Read the model definition and answer for the solid it produces. Units are mm, in the model's axes. A direction names the side the tool comes from. Coordinates: 2 decimals unless noted, no trailing zeros. Order: outer loops, then holes, each group sorted by start corner. A loop starts at its lowest first (then second) coordinate and runs counter-clockwise, first axis right, second up. Notation, with made-up numbers: M -11.75,33 L 23.25,33 A24 cw 23.25,53 Z; hole C -14.5,-18.75 d7. An arc over 180 degrees is marked long. Put each result on its own line as item: value.
from build123d import *

# Parameters (mm, degrees)
F0_R     = 1.6
F0_R_2   = 1.130501
F0_R_3   = 4.5
F0_R_4   = 5.5
F0_R_5   = 1.1305
F1_DEPTH = 1.6


with BuildPart() as f1:
    # F0 (on Top) → F1 (new body)
    with BuildSketch(Plane.XY):
        with BuildLine():
            Line((0, 6.68), (-4.5, 6.68))
            Line((-4.5, 6.68), (-4.5, 17.5))
            Line((-4.5, 17.5), (-10.717738, 23.909049))
            Line((-10.717738, 23.909049), (-12.710509, 25.963134))
            ThreePointArc((-12.710509, 25.963134), (-15.99118, 28.209543), (-19.887888, 29.000001))
            Line((-19.887888, 29.000001), (-27.5, 29.000001))
            ThreePointArc((-27.5, 29.000001), (-31.742641, 27.242641), (-33.5, 23.000001))
            Line((-33.5, 23.000001), (-33.5, 7))
            ThreePointArc((-33.5, 7), (-32.053216, 2.411389), (-28.236161, -0.517541))
            Line((-28.236161, -0.517541), (-21.823232, -2.851656))
            ThreePointArc((-21.823232, -2.851656), (-19.437572, -4.682237), (-18.533332, -7.550119))
            Line((-18.533332, -7.550119), (-18.533332, -8))
            Line((-18.533332, -8), (-18.533332, -8.449881))
            ThreePointArc((-18.533332, -8.449881), (-19.437572, -11.317763), (-21.823232, -13.148344))
            Line((-21.823232, -13.148344), (-28.236161, -15.482459))
            ThreePointArc((-28.236161, -15.482459), (-32.053216, -18.411389), (-33.5, -23))
            Line((-33.5, -23), (-33.5, -29.5))
            ThreePointArc((-33.5, -29.5), (-31.156854, -35.156854), (-25.5, -37.5))
            Line((-25.5, -37.5), (-20.777138, -37.5))
            ThreePointArc((-20.777138, -37.5), (-17.336651, -36.747083), (-14.525119, -34.625971))
            ThreePointArc((-14.525119, -34.625971), (-7.993173, -29.698059), (0, -27.94883))
            ThreePointArc((0, -27.94883), (7.993173, -29.698059), (14.525119, -34.625971))
            ThreePointArc((14.525119, -34.625971), (17.336651, -36.747083), (20.777138, -37.5))
            Line((20.777138, -37.5), (25.5, -37.5))
            ThreePointArc((25.5, -37.5), (31.156854, -35.156854), (33.5, -29.5))
            Line((33.5, -29.5), (33.5, -23))
            ThreePointArc((33.5, -23), (32.053216, -18.411389), (28.236161, -15.482459))
            Line((28.236161, -15.482459), (21.823232, -13.148344))
            ThreePointArc((21.823232, -13.148344), (19.437572, -11.317763), (18.533332, -8.449881))
            Line((18.533332, -8.449881), (18.533332, -8))
            Line((18.533332, -8), (18.533332, -7.550119))
            ThreePointArc((18.533332, -7.550119), (19.437572, -4.682237), (21.823232, -2.851656))
            Line((21.823232, -2.851656), (28.236161, -0.517541))
            ThreePointArc((28.236161, -0.517541), (32.053216, 2.411389), (33.5, 7))
            Line((33.5, 7), (33.5, 23.000001))
            ThreePointArc((33.5, 23.000001), (31.742641, 27.242641), (27.5, 29.000001))
            Line((27.5, 29.000001), (19.887888, 29.000001))
            ThreePointArc((19.887888, 29.000001), (15.99118, 28.209543), (12.710509, 25.963134))
            Line((12.710509, 25.963134), (10.717738, 23.909049))
            Line((10.717738, 23.909049), (4.5, 17.5))
            Line((4.5, 17.5), (4.5, 6.68))
            Line((4.5, 6.68), (0, 6.68))
        make_face()
        with Locations((-25.5, -33.5)):
            Circle(F0_R, mode=Mode.SUBTRACT)
        with Locations((-17.5, -30)):
            Circle(F0_R_2, mode=Mode.SUBTRACT)
        with Locations((-25.5, -23)):
            Circle(F0_R_3, mode=Mode.SUBTRACT)
        with Locations((-15.25, -23.25)):
            Circle(F0_R, mode=Mode.SUBTRACT)
        with Locations((15.25, -23.25)):
            Circle(F0_R, mode=Mode.SUBTRACT)
        with Locations((17.5, -30)):
            Circle(F0_R_2, mode=Mode.SUBTRACT)
        with Locations((25.5, -33.5)):
            Circle(F0_R, mode=Mode.SUBTRACT)
        with Locations((25.5, -23)):
            Circle(F0_R_3, mode=Mode.SUBTRACT)
        with Locations((0, -8)):
            Circle(F0_R_4, mode=Mode.SUBTRACT)
        with Locations((-25.5, 7)):
            Circle(F0_R_3, mode=Mode.SUBTRACT)
        with Locations((-15.25, 7.25)):
            Circle(F0_R, mode=Mode.SUBTRACT)
        with Locations((-25.5, 17.5)):
            Circle(F0_R, mode=Mode.SUBTRACT)
        with Locations((-17.500001, 16.5)):
            Circle(F0_R_5, mode=Mode.SUBTRACT)
        with Locations((-23.5, 24.000001)):
            Circle(F0_R_2, mode=Mode.SUBTRACT)
        with Locations((15.25, 7.25)):
            Circle(F0_R, mode=Mode.SUBTRACT)
        with Locations((25.5, 7)):
            Circle(F0_R_3, mode=Mode.SUBTRACT)
        with Locations((17.500001, 16.5)):
            Circle(F0_R_5, mode=Mode.SUBTRACT)
        with Locations((25.5, 17.5)):
            Circle(F0_R, mode=Mode.SUBTRACT)
        with Locations((23.5, 24.000001)):
            Circle(F0_R_2, mode=Mode.SUBTRACT)
    extrude(amount=F1_DEPTH)


solid = f1.part
Q1. Find section C-C on x = 15.5. Write down the section's boundary in (y, z).
Answers below:
outline: M -35.59,0 L -24.83,0 L -24.83,1.6 L -35.59,1.6 Z; M -21.67,0 L 5.67,0 L 5.67,1.6 L -21.67,1.6 Z; M 8.83,0 L 27.99,0 L 27.99,1.6 L 8.83,1.6 Z
Q2. Consider line 1 along X through (y, z) = (-26, 1.3); line 2 along X through (y, z) = (-21, 0.2); line 3 along Y through (x, z) = (15, 0.9). Determine where each line is inside the solid, lowest interval first.
Answers below:
line 1: x = -33.5 to -28.85, -22.15 to 22.15, 28.85 to 33.5
line 2: x = -33.25 to -29.53, -21.47 to 21.47, 29.53 to 33.25
line 3: y = -35.13 to -24.83, -21.67 to 5.67, 8.83 to 27.72
Q3. Find section A-A on x = -2.5. Write down the section's boundary in (y, z), plus the area to 3 significant figures.
Answers below:
outline: M -28.11,0 L -12.9,0 L -12.9,1.6 L -28.11,1.6 Z; M -3.1,0 L 6.68,0 L 6.68,1.6 L -3.1,1.6 Z
area: 40.0 mm^2
Q4. Given pin 1 (14.5 mm diameter, centred on x = -25.5, y = 7, fed in from +Z), flat-ended and moving along its own axis, determine where the tip first touches the part or whether it passes through.
Answers below:
pin 1: stops at z = 1.6
Q5. Find section B-B on y = 3.5. Write down the section's boundary in (x, z), plus the area to 3 significant figures.
Answers below:
outline: M -32.69,0 L -28.33,0 L -28.33,1.6 L -32.69,1.6 Z; M -22.67,0 L 22.67,0 L 22.67,1.6 L -22.67,1.6 Z; M 28.33,0 L 32.69,0 L 32.69,1.6 L 28.33,1.6 Z
area: 86.5 mm^2
Q6. A tool of negligible diameter and unlimited length cuts with its end or side. For faces 4 (the face through (-24.985, -14.299, 0.789)), 5 (the face through (32.014, 2.356, 0.789)), 6 (the face through (-23.745, 22.896, 0.789)), from which of +Z, -Z, +X, -X, +Y, -Y can it reach the whole face along a straight path? Write none if from no direction.
Answers below:
face 4: +Z, -Z, -X
face 5: +Z, -Z, +X
face 6: +Z, -Z
Q7. For a pull along X with two mould halves and no side action, classify faces 1 (the face through (-24, 29, 1)), 2 (the face through (25.292, 19.086, 0.789)), 3 (the face through (33.5, -26, 1)) as +X half, -X half, draft (parallel to the pull), parting line (faces both ways), or undercut.
Answers below:
face 1: draft
face 2: undercut
face 3: +X half
Q8. Find section D-D on z = 0.25. Give the number of separate pieces and of enclosed holes in the cut face, plus the area to 3 significant figures.
Answers below:
separate pieces: 1
enclosed holes: 19
area: 3,000 mm^2
